from build123d import *

# Parameters (mm, degrees)
SKETCH1_W           = 20
SKETCH1_H           = 20
BOSS_EXTRUDE1_DEPTH = 2
SKETCH2_W           = 2
SKETCH2_H           = 20
BOSS_EXTRUDE2_DEPTH = 51
SKETCH3_W           = 2
SKETCH3_H           = 20
BOSS_EXTRUDE3_DEPTH = 18
SKETCH4_R           = 2
CUT_EXTRUDE1_DEPTH  = 18
CUT_EXTRUDE2_DEPTH  = 18


with BuildPart() as part:
    # Sketch1 → Boss-Extrude1 (new body)
    with BuildSketch(Plane.XY):
        Rectangle(SKETCH1_W, SKETCH1_H)
    extrude(amount=BOSS_EXTRUDE1_DEPTH)

    # Sketch2 → Boss-Extrude2 (add)
    with BuildSketch(Plane.XY.offset(2)):
        with Locations((-9, 0)):
            Rectangle(SKETCH2_W, SKETCH2_H)
    extrude(amount=BOSS_EXTRUDE2_DEPTH)

    # Sketch3 → Boss-Extrude3 (add)
    with BuildSketch(Plane(origin=(-8, 0, 0), x_dir=(0, 0, -1), z_dir=(1, 0, 0))):
        with Locations((-52, 0)):
            Rectangle(SKETCH3_W, SKETCH3_H)
    extrude(amount=BOSS_EXTRUDE3_DEPTH)

    # Sketch4 → Cut-Extrude1 (cut)
    with BuildSketch(Plane.XY.offset(53)):
        Circle(SKETCH4_R)
    extrude(amount=-CUT_EXTRUDE1_DEPTH, mode=Mode.SUBTRACT)

    # Sketch5 → Cut-Extrude2 (cut)
    with BuildSketch(Plane(origin=(0, 0, 0), x_dir=(-1, 0, 0), z_dir=(0, 0, -1))):
        with BuildLine():
            Line((-6, 2), (4, 2))
            ThreePointArc((4, 2), (6, 0), (4, -2))
            Line((4, -2), (-6, -2))
            ThreePointArc((-6, -2), (-8, 0), (-6, 2))
        make_face()
    extrude(amount=-CUT_EXTRUDE2_DEPTH, mode=Mode.SUBTRACT)


solid = part.part
Check sheet for the modelled part. Datum: model origin and axes. Units: mm. A direction names the side the tool comes from. Give positions to 0.01 mm unless a question says otherwise; leave off trailing zeros. Order: outer loops, then holes, each group sorted by start corner. A loop starts at its lowest first (then second) coordinate and runs counter-clockwise, first axis right, second up. Notation, with made-up numbers: (24.5, 4) - (47.5, 4) arc R22 ccw to (47.5, 19) - close; hole circle Ø2 at (-23.5, 82). An arc over 180 degrees is marked (long way). Answer as CSV lines item,"result".
1. Section check B-B (x = 8.5). Record the boundary of the cut face in (y, z).
Result sheet:
outline,"(-10, 0) - (10, 0) - (10, 2) - (-10, 2) - close; (-10, 51) - (10, 51) - (10, 53) - (-10, 53) - close"
2. Section check A-A (y = 0). Record the boundary of the cut face in (x, z), then the cut area to 3 significant figures.
Result sheet:
outline,"(-10, 0) - (-6, 0) - (-6, 2) - (-8, 2) - (-8, 51) - (-2, 51) - (-2, 53) - (-10, 53) - close; (2, 51) - (10, 51) - (10, 53) - (2, 53) - close; (8, 0) - (10, 0) - (10, 2) - (8, 2) - close"
area,"142 mm²"
3. Mould release check, pull along Z, two halves, no side actions. Record for faces 4 (the face through (1, 2, 1)), 5 (the face through (-2.4, -0.1, 53)), 6 (the face through (0.9, 2.4, 2)), 7 (the face through (-0.1, 2.4, 0)): released by +Z, released by -Z, zero draft, split by the parting line, or undercut.
Result sheet:
face 4,"zero draft"
face 5,"released by +Z"
face 6,"undercut"
face 7,"released by -Z"
4. Scan lines: probe 1 along Z at (x, y) = (8.25, -4.75); probe 2 along Y at (x, z) = (0, 52.5); probe 3 along X at (y, z) = (4.25, 48). Record each from-to range of solid material in increasing order. Write a range as from..to.
Result sheet:
probe 1,"0..2, 51..53"
probe 2,"-10..-2, 2..10"
probe 3,"-10..-8"
5. Section check D-D (y = -7). Record the boundary of the cut face in (x, z).
Result sheet:
outline,"(-10, 0) - (10, 0) - (10, 2) - (-8, 2) - (-8, 51) - (10, 51) - (10, 53) - (-10, 53) - close"
6. Section check C-C (x = -2.5). Record the boundary of the cut face in (y, z).
Result sheet:
outline,"(-10, 0) - (-2, 0) - (-2, 2) - (-10, 2) - close; (-10, 51) - (10, 51) - (10, 53) - (-10, 53) - close; (2, 0) - (10, 0) - (10, 2) - (2, 2) - close"
7. Tool access check on faces 1 (the face through (-8.2, 10, 26.6)), 2 (the face through (3, 0, 51)), 3 (the face through (-6, 0, 1)). Record the directions out of +Z, -Z, +X, -X, +Y, -Y that give a thin tool (end or side, any length) a straight path to the whole face; none if there is none.
Result sheet:
face 1,"+Z, -Z, +X, -X, +Y"
face 2,"+X, +Y, -Y"
face 3,"-Z"
8. Go/stop test with flat-tipped pins: P1, Ø3, axis at x = 2.5, y = 1.5, coming from the -Z side; P2, Ø10, axis at y = 2.5, z = 22.5, coming from the +X side; P3, Ø6, axis at x = -3.5, z = 14, coming from the -Y side. Record where each tip stops, or that it passes through.
Result sheet:
P1,"z = 0"
P2,"x = -8"
P3,"through"
